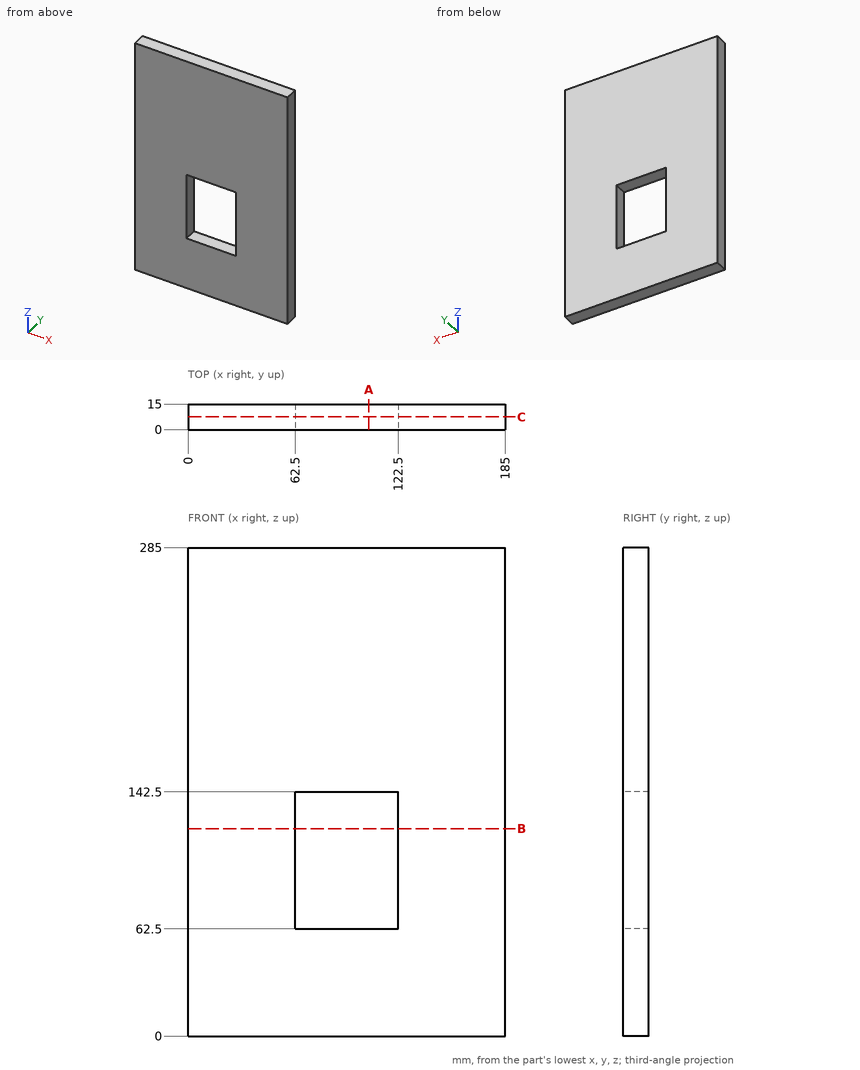
Verification items for this drawing (mm, ordinates from the low corner). Coordinates: 2 decimals unless noted, no trailing zeros. Loops run counter-clockwise (first coordinate to the right, second up) from the corner with the lowest first, then second, coordinate; pieces in that order, holes last. Notation, with made-up numbers: (-26.5, 24) -> (14.5, 24) arc R27 cw to (14.5, 56) -> close; hole circle Ø7 at (39, 13.5). An arc over 180 degrees is marked (long way). Answer in a Markdown table with one row per item. Add a question column.
1. Section check A-A, the plane x = 105.5. Enter the section's corners in (y, z).
2. Section check B-B, the plane z = 121. Enter the section's corners in (x, y), then the cut area to 4 significant figures.
3. Section check C-C, the plane y = 7.5. Enter the section's corners in (x, z).
4. Material ranges on probe 1 along Z at (x, y) = (98, 3); probe 2 along X at (y, z) = (13, 89), recorded low to high. Write a range as [from, to].
Derived:
| question | item | result |
|---|---|---|
| 1 | outline | (0, 0) -> (15, 0) -> (15, 62.5) -> (0, 62.5) -> close; (0, 142.5) -> (15, 142.5) -> (15, 285) -> (0, 285) -> close |
| 2 | outline | (0, 0) -> (62.5, 0) -> (62.5, 15) -> (0, 15) -> close; (122.5, 0) -> (185, 0) -> (185, 15) -> (122.5, 15) -> close |
| 2 | area | 1,875 mm² |
| 3 | outline | (0, 0) -> (185, 0) -> (185, 285) -> (0, 285) -> close; hole (62.5, 62.5) -> (122.5, 62.5) -> (122.5, 142.5) -> (62.5, 142.5) -> close |
| 4 | probe 1 | z = [0, 62.5], [142.5, 285] |
| 4 | probe 2 | x = [0, 62.5], [122.5, 185] |
